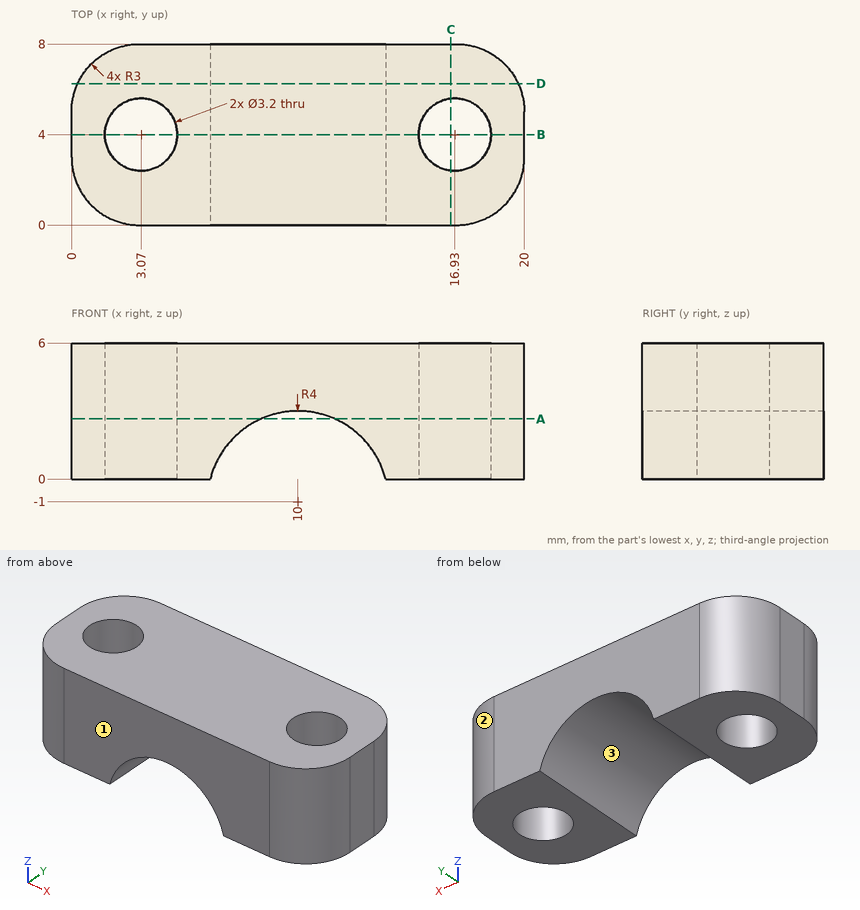
Could you check a few things on this drawing? It's one solid part, dimensions in mm from its lowest x, y, z. Coordinates: 2 decimals unless noted, no trailing zeros. Loops run counter-clockwise (first coordinate to the right, second up) from the corner with the lowest first, then second, coordinate; pieces in that order, holes last. Notation, with made-up numbers: (26.5, -25.75) - (54.5, -25.75) arc R10 cw to (54.5, -14.75) - close; hole circle Ø1 at (9.5, 68). An arc over 180 degrees is marked (long way). Return JSON: item names as keys, results as strings. Group by question number.
Item 1: We'd pull the mould along X, two halves only. Please class the marked faces 1, 2 and 3: +X half, -X half, draft (parallel to the pull), parting line (faces both ways), or undercut.
Item 2: If we section it at B-B on y = 4: Write out the boundary of the cut face in (x, z).
Item 3: If we section it at D-D on y = 6.25: Write out the boundary of the cut face in (x, z), and give its area (3 significant figures).
Item 4: If we section it at C-C on x = 16.75: Write out the boundary of the cut face in (y, z), and give its area (3 significant figures).
Item 5: If we section it at A-A on z = 2.65: Write out the boundary of the cut face in (x, y), and give its area (3 significant figures).
Item 6: I need wall thicknesses on line 1 (X direction, y = 4, z = 3.8); line 2 (Y direction, x = 16.93, z = 1.3); line 3 (X direction, y = 4, z = 1.3). Which ranges of each line are inside material? Lowest first, please. Write a range as from..to.
Calculated:
{
 "1": {"face 1": "draft", "face 2": "+X half", "face 3": "undercut"},
 "2": {"outline": "(0, 0) - (1.47, 0) - (1.47, 6) - (0, 6) - close; (4.67, 0) - (6.13, 0) arc R4 cw to (13.87, 0) - (15.33, 0) - (15.33, 6) - (4.67, 6) - close; (18.53, 0) - (20, 0) - (20, 6) - (18.53, 6) - close"},
 "3": {"outline": "(0.27, 0) - (6.13, 0) arc R4 cw to (13.87, 0) - (19.73, 0) - (19.73, 6) - (0.27, 6) - close", "area": "99.5 mm^2"},
 "4": {"outline": "(0, 0) - (2.41, 0) - (2.41, 6) - (0, 6) - close; (5.59, 0) - (8, 0) - (8, 6) - (5.59, 6) - close", "area": "28.9 mm^2"},
 "5": {"outline": "(0, 3) arc R3 ccw to (3, 0) - (8.36, 0) - (8.36, 8) - (3, 8) arc R3 ccw to (0, 5) - close; (11.64, 0) - (17, 0) arc R3 ccw to (20, 3) - (20, 5) arc R3 ccw to (17, 8) - (11.64, 8) - close; hole circle Ø3.2 at (3.07, 4); hole circle Ø3.2 at (16.93, 4)", "area": "110 mm^2"},
 "6": {"line 1": "x = 0..1.47, 4.67..15.33, 18.53..20", "line 2": "y = 0..2.4, 5.6..8", "line 3": "x = 0..1.47, 4.67..6.73, 13.27..15.33, 18.53..20"}
}
